```python
from build123d import *

# Parameters (mm, degrees)
F1_DEPTH       = 10
F3_D           = 9
F3_CSINK_D     = 16.4
F3_CSINK_ANGLE = 90
F4_D           = 6.5
F4_CBORE_D     = 11
F4_CBORE_DEPTH = 6.4


with BuildPart() as f1:
    # F0 (on Top) → F1 (new body)
    with BuildSketch(Plane.XY):
        with BuildLine():
            Line((0, 20), (20, 0))
            Line((20, 0), (80, 0))
            Line((80, 0), (80, 60))
            Line((80, 60), (66.5, 60))
            ThreePointArc((66.5, 60), (62.232233, 58.232233), (64, 62.5))
            Line((64, 62.5), (64, 80))
            Line((64, 80), (0, 80))
            Line((0, 80), (0, 20))
        make_face()
    extrude(amount=F1_DEPTH)

    # F3 (through all)
    with Locations(Plane.XY.offset(10)):
        with Locations((64, 20)):
            CounterSinkHole(F3_D / 2, F3_CSINK_D / 2, counter_sink_angle=F3_CSINK_ANGLE)

    # F4 (through all)
    with Locations(Plane.XY.offset(10)):
        with Locations((64, 40)):
            CounterBoreHole(F4_D / 2, F4_CBORE_D / 2, F4_CBORE_DEPTH)


solid = f1.part
```
Check sheet for the modelled part. Datum: model origin and axes. Units: mm. A direction names the side the tool comes from. Round coordinates to 2 decimals unless told otherwise and drop trailing zeros. Order: outer loops, then holes, each group sorted by start corner. A loop starts at its lowest first (then second) coordinate and runs counter-clockwise, first axis right, second up. Notation, with made-up numbers: (-38, -13) - (12, -13) arc R31 ccw to (12, 26) - close; hole circle Ø4 at (-2.75, -10). An arc over 180 degrees is marked (long way). Answer as CSV lines item,"result". Start each with the question number.
1) Draft check along X on faces 1 (the face through (61.581, 23.794, 3.106)), 2 (the face through (0, 50, 5)), 3 (the face through (39, 41, 0)). Enter one of: +X half, -X half, draft (parallel to the pull), parting line (faces both ways), or undercut.
2) Section check B-B (z = 1.25). Record the cut outline in (x, y), then the cut area to 3 significant figures.
3) Depth check by flat-ended pin: pin 1 (3 mm diameter, centred on y = 72, z = 6.5, fed in from +X); pin 2 (5.5 mm diameter, centred on x = 64.5, y = 38.5, fed in from +Z); pin 3 (5 mm diameter, centred on x = 76, z = 5, fed in from +Y). Enter the tip coordinate at first touch or a pass-through.
4) Scan lines: probe 1 along X at (y, z) = (20, 2.75); probe 2 along Y at (x, z) = (60, 7.25); probe 3 along X at (y, z) = (62, 6.25). Record each from-to range of solid material in increasing order.
5) Tool access check on faces 4 (the face through (58.505, 40.242, 6.845)), 5 (the face through (66.579, 38.022, 1.775)), 6 (the face through (64, 71, 5)). Record the directions out of +Z, -Z, +X, -X, +Y, -Y that give a thin tool (end or side, any length) a straight path to the whole face; none if there is none.
6) Section check C-C (z = 7.75). Record the cut outline in (x, y).
7) Section check D-D (y = 7.5). Record the cut outline in (x, z), then the cut area to 3 significant figures.
8) Section check A-A (y = 40). Record the cut outline in (x, z), then the cut area to 3 significant figures.
Determined:
1,face 1,"undercut"
1,face 2,"-X half"
1,face 3,"draft"
2,outline,"(0, 20) - (20, 0) - (80, 0) - (80, 60) - (66.5, 60) arc R2.5 cw (long way) to (64, 62.5) - (64, 80) - (0, 80) - close; hole circle Ø9 at (64, 20); hole circle Ø6.5 at (64, 40)"
2,area,"5,770 mm^2"
3,pin 1,"x = 64"
3,pin 2,"z = 3.6"
3,pin 3,"y = 60"
4,probe 1,"0 to 59.5, 68.5 to 80"
4,probe 2,"0 to 16.3, 23.7 to 36.23, 43.77 to 80"
4,probe 3,"0 to 62.5"
5,face 4,"+Z"
5,face 5,"+Z, -Z"
5,face 6,"+Z, -Z, +X, +Y"
6,outline,"(0, 20) - (20, 0) - (80, 0) - (80, 60) - (66.5, 60) arc R2.5 cw (long way) to (64, 62.5) - (64, 80) - (0, 80) - close; hole circle Ø11.9 at (64, 20); hole circle Ø11 at (64, 40)"
7,outline,"(12.5, 0) - (80, 0) - (80, 10) - (12.5, 10) - close"
7,area,"675 mm^2"
8,outline,"(0, 0) - (60.75, 0) - (60.75, 3.6) - (58.5, 3.6) - (58.5, 10) - (0, 10) - close; (67.25, 0) - (80, 0) - (80, 10) - (69.5, 10) - (69.5, 3.6) - (67.25, 3.6) - close"
8,area,"706 mm^2"
